from build123d import *

# Parameters (mm, degrees)
F0_R     = 2.4
F1_DEPTH = 1.8
F2_R     = 3.9
F2_R_2   = 2.4
F3_DEPTH = 9.6
F4_R     = 3.9
F4_R_2   = 3.2
F5_DEPTH = 1.8
F6_R     = 2.3
F7_DEPTH = 8.8
F8_R     = 1.6
F9_DEPTH = 1.8


# Not quite as in the source:
# - a feature names something its author has since deleted; it is built from what else it names


with BuildPart() as f1:
    # F0 (on Top) → F1 (new body)
    with BuildSketch(Plane.XY):
        Circle(F0_R)
    extrude(amount=F1_DEPTH)

    # F2 (on face) → F3 (join)
    with BuildSketch(Plane.XY.offset(1.8)):
        Circle(F2_R)
        Circle(F2_R_2, mode=Mode.SUBTRACT)
        Circle(F2_R_2)
    extrude(amount=F3_DEPTH)

    # F4 (on face) → F5 (cut)
    with BuildSketch(Plane.XY.offset(11.4)):
        Circle(F4_R)
        Circle(F4_R_2, mode=Mode.SUBTRACT)
    extrude(amount=-F5_DEPTH, mode=Mode.SUBTRACT)

    # F6 (on face) → F7 (cut)
    with BuildSketch(Plane.XY.offset(11.4)):
        Circle(F6_R)
    extrude(amount=-F7_DEPTH, mode=Mode.SUBTRACT)

    # F8 (on face) → F9 (cut)
    with BuildSketch(Plane.XY.offset(2.6)):
        Circle(F8_R)
    extrude(amount=-F9_DEPTH, mode=Mode.SUBTRACT)


solid = f1.part
Input: part model. Units: mm. Frame: model coordinates. A direction names the side the tool comes from. Give positions to 0.01 mm unless a question says otherwise; leave off trailing zeros. Order: outer loops, then holes, each group sorted by start corner. A loop starts at its lowest first (then second) coordinate and runs counter-clockwise, first axis right, second up. Notation, with made-up numbers: (-31.5, -36) - (8.5, -36) arc R38 cw to (8.5, 2) - close; hole circle Ø7 at (-16, -18.5). An arc over 180 degrees is marked (long way). Answer as a JSON object with one key per item and string values. Group by question number.
Q1. Cut plane D-D, the plane x = -2. Output: boundary loops of the cut face in (y, z), then the cut area to 3 significant figures.
Q2. Cut plane B-B, the plane z = 4.5. Output: boundary loops of the cut face in (x, y).
Q3. Line query: probe 1 along Y at (x, z) = (0, 8); probe 2 along Y at (x, z) = (0, 1.6); probe 3 along X at (y, z) = (1.5, 5.5). Output: solid intervals per line, ascending.
Q4. First-contact query: pin 1 Ø1 at (x, y) = (0.5, -0.5) entering from +Z; pin 2 Ø1 at (y, z) = (2, 3.5) entering from -X; pin 3 Ø1 at (x, z) = (1.5, 6.5) entering from +Y. Flat tips, straight axial feed; report the tip coordinate or a pass-through.
Q5. Mould query, pull axis Y, two halves, no side actions, for faces 1 (the face through (-2.87, 2.64, 5.65)), 2 (the face through (0, 0, 0)), 3 (the face through (-2, 0, 2.6)), 4 (the face through (-1.825, -1.4, 7.062)). Classes: pulls with the +Y half, pulls with the -Y half, needs draft (parallel to the pull), parting line crosses it, or undercut.
Q6. Set-up query: faces 5 (the face through (1.29, 2.024, 0.887)), 6 (the face through (2.1, -1.4, 11.4)), 7 (the face through (-1.27, -0.97, 1.71)). Return all of +Z, -Z, +X, -X, +Y, -Y with unobstructed straight access to the full face (end or side cutting, diameter ignored); none if empty.
Q7. Cut plane A-A, the plane x = 0. Output: boundary loops of the cut face in (y, z), then the cut area to 3 significant figures.
Results:
{
 "1": {"outline": "(-3.35, 1.8) - (-1.33, 1.8) - (-1.33, 0) - (1.33, 0) - (1.33, 1.8) - (3.35, 1.8) - (3.35, 9.6) - (2.5, 9.6) - (2.5, 11.4) - (1.14, 11.4) - (1.14, 2.6) - (-1.14, 2.6) - (-1.14, 11.4) - (-2.5, 11.4) - (-2.5, 9.6) - (-3.35, 9.6) - close", "area": "46.0 mm^2"},
 "2": {"outline": "circle Ø7.8 at (0, 0); hole circle Ø4.6 at (0, 0)"},
 "3": {"probe 1": "-3.9 to -2.3, 2.3 to 3.9", "probe 2": "-2.4 to -1.6, 1.6 to 2.4", "probe 3": "-3.6 to -1.74, 1.74 to 3.6"},
 "4": {"pin 1": "z = 0.8", "pin 2": "x = -3.6", "pin 3": "y = 3.77"},
 "5": {"face 1": "parting line crosses it", "face 2": "needs draft", "face 3": "undercut", "face 4": "undercut"},
 "6": {"face 5": "-Z", "face 6": "+Z, +X, -X, +Y, -Y", "face 7": "+Z"},
 "7": {"outline": "(-3.9, 1.8) - (-2.4, 1.8) - (-2.4, 0) - (2.4, 0) - (2.4, 1.8) - (3.9, 1.8) - (3.9, 9.6) - (3.2, 9.6) - (3.2, 11.4) - (2.3, 11.4) - (2.3, 2.6) - (1.6, 2.6) - (1.6, 0.8) - (-1.6, 0.8) - (-1.6, 2.6) - (-2.3, 2.6) - (-2.3, 11.4) - (-3.2, 11.4) - (-3.2, 9.6) - (-3.9, 9.6) - close", "area": "34.8 mm^2"}
}
